Read the model definition and answer for the solid it produces. Units are mm, in the model's axes. A direction names the side the tool comes from. Coordinates: 2 decimals unless noted, no trailing zeros. Loops run counter-clockwise (first coordinate to the right, second up) from the corner with the lowest first, then second, coordinate; pieces in that order, holes last. Notation, with made-up numbers: (-10.75, -30.5) -> (35.25, -30.5) arc R19 cw to (35.25, -20.5) -> close; hole circle Ø4 at (19, 18). An arc over 180 degrees is marked (long way). Answer as a JSON object with one key per item and string values. Group by question number.
Q1. Straight lines are drawn through the part: line 1 along Z through (x, y) = (0, -53); line 2 along X through (y, z) = (-53, 3); line 3 along Z through (x, y) = (0, -25). For each, find the intervals that lie inside material, in ascending order. Write a range as [from, to].
Q2. The part is cut by section C-C on y = -15.5. Write down the section's boundary in (x, z), and give its area (3 significant figures).
Q3. The part is cut by section D-D on x = 7. Write down the section's boundary in (y, z).
Q4. The part is cut by section B-B on y = -28. Write down the section's boundary in (x, z), and give its area (3 significant figures).
Q5. For faces 4 (the cylindrical face through (12.4, -39.4, 3.9)), 5 (the flat face through (16, -33, -3)), 6 (the flat face through (0, -42, 19)), determine the directions among +Z, -Z, +X, -X, +Y, -Y from which every point of the face is accessible in a straight line to the end or side of a thin tool.
Q6. Determine the mould class of faces 1 (the cylindrical face through (17.089, -20.706, 7.086)), 2 (the flat face through (0, 20, 0)), 3 (the flat face through (-16, -20, 0)) for opening direction Z: released by +Z, released by -Z, zero draft, split by the parting line, or undercut.
Q7. The part is cut by section A-A on z = 0. Write down the section's boundary in (x, y).
Q8. Each of these flat-tipped pins is pushed along its axis until it touches: P1, Ø9.5, axis at x = 21, y = -33, coming from the -Z side; P2, Ø1.8, axis at x = 18, z = 0, coming from the +Y side; P3, Ø6, axis at x = -19, y = -33.5, coming from the -Z side. Where does it stop, or does it pass through?
Solid Edge part; units mm, degrees
sketch "Sketch1" plane through (0, 0, 0) normal (0, -1, 0) x (1, 0, 0)
  circle A0 centre (0, 0) radius 10
extrude "Protrusion1" add sketch "Sketch1" against normal blind 20
sketch "Sketch2" plane through (0, 0, 0) normal (0, -1, 0) x (1, 0, 0)
  circle A0 centre (0, 0) radius 18.5
extrude "ExtrudedProtrusion_2" add sketch "Sketch2" along normal blind 42
sketch "Sketch3" plane through (0, -42, 0) normal (0, -1, 0) x (1, 0, 0)
  circle A0 centre (0, 0) radius 25
extrude "ExtrudedProtrusion_3" add sketch "Sketch3" along normal blind 24
sketch "Sketch4" plane through (0, -66, 0) normal (0, -1, 0) x (1, 0, 0)
  circle A0 centre (0, 0) radius 13
extrude "ExtrudedCutout_1" cut sketch "Sketch4" against normal blind 54
sketch "Sketch5" plane through (0, 0, 0) normal (1, 0, 0) x (0, 1, 0)
  line L0 (-46, 3) -> (-20, 3)
  line L1 (-20, 3) -> (-20, -3)
  line L2 (-20, -3) -> (-46, -3)
  line L3 (-46, -3) -> (-46, 3)
  dimension "D1" = 46
  dimension "D2" = 46
extrude "ExtrudedCutout_2" cut sketch "Sketch5" along normal mid plane 185.6851
properties part number "1"
Final values:
{
 "1": {"line 1": "z = [-25, -13], [13, 25]", "line 2": "x = [-24.82, -12.65], [12.65, 24.82]", "line 3": "z = [-18.5, -13], [13, 18.5]"},
 "2": {"outline": "circle Ø37 at (0, 0); hole circle Ø26 at (0, 0)", "area": "544 mm2"},
 "3": {"outline": "(-66, -24) -> (-42, -24) -> (-42, -17.12) -> (0, -17.12) -> (0, -7.14) -> (20, -7.14) -> (20, 7.14) -> (0, 7.14) -> (0, 17.12) -> (-42, 17.12) -> (-42, 24) -> (-66, 24) -> (-66, 10.95) -> (-12, 10.95) -> (-12, -10.95) -> (-66, -10.95) -> close"},
 "4": {"outline": "(-18.26, -3) arc R18.5 ccw to (18.26, -3) -> (12.65, -3) arc R13 cw to (-12.65, -3) -> close; (-18.26, 3) -> (-12.65, 3) arc R13 cw to (12.65, 3) -> (18.26, 3) arc R18.5 ccw to start", "area": "478 mm2"},
 "5": {"face 4": "-Y", "face 5": "+X, -X", "face 6": "+Z, +Y"},
 "6": {"face 1": "split by the parting line", "face 2": "zero draft", "face 3": "undercut"},
 "7": {"outline": "(-25, -66) -> (-13, -66) -> (-13, -46) -> (-25, -46) -> close; (-18.5, -20) -> (-13, -20) -> (-13, -12) -> (13, -12) -> (13, -20) -> (18.5, -20) -> (18.5, 0) -> (10, 0) -> (10, 20) -> (-10, 20) -> (-10, 0) -> (-18.5, 0) -> close; (13, -66) -> (25, -66) -> (25, -46) -> (13, -46) -> close"},
 "8": {"P1": "stops at z = -8.84", "P2": "stops at y = 0", "P3": "stops at z = -9.29"}
}
